Here's how the part is built. I have some questions about the finished solid (model axes, mm). A direction names the side the tool comes from. Coordinates: 2 decimals unless noted, no trailing zeros. Write each loop counter-clockwise with the first axis right and the second up, starting at its lowest first coordinate (ties: lowest second). Pieces come first, ordered by that corner, then holes.
from build123d import *

# Parameters (mm, degrees)
SKETCH_W       = 15.88
SKETCH_H       = 44.46
SKETCH_R       = 2.775
PAD_DEPTH      = 4.4
PAD_FACE1_W    = 4.4
PAD_FACE1_H    = 15.88
PAD001_DEPTH   = 4.4
PAD001_FACE6_W = 15.88
PAD001_FACE6_H = 4.4
PAD002_DEPTH   = 50
PAD002_FACE7_W = 15.88
PAD002_FACE7_H = 4.4
PAD003_DEPTH   = 25


with BuildPart() as part:
    # Sketch → Pad (new body)
    with BuildSketch(Plane.XZ):
        with Locations((7.94, 22.23)):
            Rectangle(SKETCH_W, SKETCH_H)
        with Locations((7.874, 6.35)):
            Circle(SKETCH_R, mode=Mode.SUBTRACT)
        with Locations((7.874, 22.23)):
            Circle(SKETCH_R, mode=Mode.SUBTRACT)
        with Locations((7.874, 38.11)):
            Circle(SKETCH_R, mode=Mode.SUBTRACT)
    extrude(amount=PAD_DEPTH)

    # Pad Face1 → Pad001 (add)
    with BuildSketch(Plane(origin=(7.94, -2.2, 0), x_dir=(0, -1, 0), z_dir=(0, 0, -1))):
        Rectangle(PAD_FACE1_W, PAD_FACE1_H)
    extrude(amount=PAD001_DEPTH)

    # Pad001 Face6 → Pad002 (add)
    with BuildSketch(Plane(origin=(7.94, 0, -2.2), x_dir=(1, 0, 0), z_dir=(0, 1, 0))):
        Rectangle(PAD001_FACE6_W, PAD001_FACE6_H)
    extrude(amount=PAD002_DEPTH)

    # Pad002 Face7 → Pad003 (add)
    with BuildSketch(Plane(origin=(7.94, -4.4, -2.2), x_dir=(-1, 0, 0), z_dir=(0, -1, 0))):
        Rectangle(PAD002_FACE7_W, PAD002_FACE7_H)
    extrude(amount=PAD003_DEPTH)


solid = part.part
1. On a 3-axis mill with a long thin cutter (end or side, diameter ignored), from which of +Z, -Z, +X, -X, +Y, -Y can I reach the whole of each face in a straight line? I mean faces 5 (the face through (8, 25, 0)), 6 (the face through (8, 50, -2)). Say none if no direction works.
2. I want a section at C-C (z = 30.5). List the corners of the cut face in (x, y) for me, then the cut area to 3 significant figures.
3. If I drill on line 1 (X direction, y = -2, z = 22); line 2 (Y direction, x = 13.75, z = 41), over which ranges is the centre line in solid material (lowest first)?
4. I want a section at A-A (z = 38.11). List the corners of the cut face in (x, y) for me.
5. I want a section at B-B (x = 4). List the corners of the cut face in (y, z) for me.
6. Thinking about a two-plate mould opening in Z: for faces 1 (the face through (10.52, -2.17, 7.18)), 2 (the face through (5, -4.4, 23)), 3 (the face through (8, -17, 0)), 4 (the face through (9.366, -2.169, 40.45)), which applies, pulls with the +Z half, pulls with the -Z half, needs draft (parallel to the pull), parting line crosses it, or undercut?
7. For pin 1 Ø1 at (x, z) = (6, 1) entering from +Y; pin 2 Ø9 at (x, z) = (7.874, 38.11) entering from -Y; pin 3 Ø5 at (x, y) = (11, 37.5) entering from +Z, each with a flat end and sliding along its axis, tell me the tip position at first contact or that it passes through.
Response values:
1. face 5: +Z, +X, -X, +Y
1. face 6: +Z, -Z, +X, -X, +Y
2. outline: (0, -4.4) - (15.88, -4.4) - (15.88, 0) - (0, 0) - close
2. area: 69.9 mm2
3. line 1: x = 0 to 5.11, 10.64 to 15.88
3. line 2: y = -4.4 to 0
4. outline: (0, -4.4) - (5.1, -4.4) - (5.1, 0) - (0, 0) - close; (10.65, -4.4) - (15.88, -4.4) - (15.88, 0) - (10.65, 0) - close
5. outline: (-29.4, -4.4) - (50, -4.4) - (50, 0) - (0, 0) - (0, 44.46) - (-4.4, 44.46) - (-4.4, 0) - (-29.4, 0) - close
6. face 1: undercut
6. face 2: needs draft
6. face 3: pulls with the +Z half
6. face 4: undercut
7. pin 1: stops at y = 0
7. pin 2: stops at y = -4.4
7. pin 3: stops at z = 0
